from build123d import *

# Parameters (mm, degrees)
SKETCH1_R           = 52.3621
BOSS_EXTRUDE1_DEPTH = 7.06
SKETCH4_R           = 1.7653
SKETCH6_R           = 1.575
CUT_EXTRUDE1_DEPTH  = 7.06
BOSS_EXTRUDE2_DEPTH = 7.06
CUT_EXTRUDE3_DEPTH  = 7.06
CHAMFER17_SIZE      = 4
CHAMFER17_SIZE2     = 2.800830153
CHAMFER18_SIZE      = 4
CHAMFER18_SIZE2     = 2.800830153
CHAMFER19_SIZE      = 4
CHAMFER19_SIZE2     = 2.800830153
CHAMFER20_SIZE      = 4
CHAMFER20_SIZE2     = 2.800830153
CHAMFER21_SIZE      = 4
CHAMFER21_SIZE2     = 2.800830153
CHAMFER25_SIZE      = 4
CHAMFER25_SIZE2     = 2.800830153
CHAMFER26_SIZE      = 4
CHAMFER26_SIZE2     = 2.800830153
CHAMFER39_SIZE      = 4
CHAMFER39_SIZE2     = 2.800830153
CHAMFER40_SIZE      = 4
CHAMFER40_SIZE2     = 2.800830153
CHAMFER42_SIZE      = 4
CHAMFER42_SIZE2     = 2.800830153
CHAMFER43_SIZE      = 4
CHAMFER43_SIZE2     = 2.800830153
CHAMFER44_SIZE      = 4
CHAMFER44_SIZE2     = 2.800830153
CHAMFER45_SIZE      = 4
CHAMFER45_SIZE2     = 2.800830153
CHAMFER46_SIZE      = 4
CHAMFER46_SIZE2     = 2.800830153


with BuildPart() as part:
    # Sketch1 → Boss-Extrude1 (new body)
    with BuildSketch(Plane(origin=(0, 0, 0), x_dir=(1, 0, 0), z_dir=(0, 1, 0))):
        with Locations(Location((0, 0, 0), (0, 0, 270))):
            Circle(SKETCH1_R)
    extrude(amount=BOSS_EXTRUDE1_DEPTH)

    # Sketch4 → Cut-Revolve2 (revolve, cut)
    with BuildSketch(Plane(origin=(0, 0, 0), x_dir=(0, 0, -1), z_dir=(1, 0, 0)), mode=Mode.PRIVATE) as cut_revolve2_sk:
        with Locations((-52.3621, 3.53)):
            Circle(SKETCH4_R)
    revolve(cut_revolve2_sk.sketch.rotate(Axis((0, 3.53, 0), (0, 1, 0)), 180), axis=Axis((0, 3.53, 0), (0, 1, 0)), mode=Mode.SUBTRACT)

    # Sketch6 → Cut-Extrude1 (cut)
    with BuildSketch(Plane(origin=(0, 7.06, 0), x_dir=(1, 0, 0), z_dir=(0, 1, 0))):
        with Locations(Location((0, 0, 0), (0, 0, 270))):
            Circle(SKETCH6_R)
    extrude(amount=-CUT_EXTRUDE1_DEPTH, mode=Mode.SUBTRACT)

    # Sketch7 → Boss-Extrude2 (add)
    with BuildSketch(Plane(origin=(0, 7.06, 0), x_dir=(1, 0, 0), z_dir=(0, 1, 0))):
        with BuildLine():
            Line((-1.173935688, 1.05), (1.173935688, 1.05))
            ThreePointArc((1.173935688, 1.05), (0, 1.575), (-1.173935688, 1.05))
        make_face()
    extrude(amount=-BOSS_EXTRUDE2_DEPTH)

    # Sketch8 → Cut-Extrude3 (cut)
    with BuildSketch(Plane(origin=(0, 7.06, 0), x_dir=(1, 0, 0), z_dir=(0, 1, 0))):
        with BuildLine():
            Line((-44.72135955, 5), (-17.291616466, 5))
            ThreePointArc((-17.291616466, 5), (-16.629831585, 6.888301783), (-15.762553167, 8.691485355))
            Line((-15.762553167, 8.691485355), (-35.158310508, 28.087242696))
            ThreePointArc((-35.158310508, 28.087242696), (-41.574578963, 17.220754456), (-44.72135955, 5))
        make_face()
        with BuildLine():
            Line((-17.291616466, -5), (-44.72135955, -5))
            ThreePointArc((-44.72135955, -5), (-41.574578963, -17.220754456), (-35.158310508, -28.087242696))
            Line((-35.158310508, -28.087242696), (-15.762553167, -8.691485355))
            ThreePointArc((-15.762553167, -8.691485355), (-16.629831585, -6.888301783), (-17.291616466, -5))
        make_face()
        with BuildLine():
            Line((17.291616466, -5), (44.72135955, -5))
            ThreePointArc((44.72135955, -5), (41.574578963, -17.220754456), (35.158310508, -28.087242696))
            Line((35.158310508, -28.087242696), (15.762553167, -8.691485355))
            ThreePointArc((15.762553167, -8.691485355), (16.629831585, -6.888301783), (17.291616466, -5))
        make_face()
        with BuildLine():
            Line((15.762553167, 8.691485355), (35.158310508, 28.087242696))
            ThreePointArc((35.158310508, 28.087242696), (41.574578963, 17.220754456), (44.72135955, 5))
            Line((44.72135955, 5), (17.291616466, 5))
            ThreePointArc((17.291616466, 5), (16.629831585, 6.888301783), (15.762553167, 8.691485355))
        make_face()
        with BuildLine():
            Line((-28.087242696, 35.158310508), (-8.691485355, 15.762553167))
            ThreePointArc((-8.691485355, 15.762553167), (-6.888301783, 16.629831585), (-5, 17.291616466))
            Line((-5, 17.291616466), (-5, 44.72135955))
            ThreePointArc((-5, 44.72135955), (-17.220754456, 41.574578963), (-28.087242696, 35.158310508))
        make_face()
        with BuildLine():
            Line((5, 17.291616466), (5, 44.72135955))
            ThreePointArc((5, 44.72135955), (17.220754456, 41.574578963), (28.087242696, 35.158310508))
            Line((28.087242696, 35.158310508), (8.691485355, 15.762553167))
            ThreePointArc((8.691485355, 15.762553167), (6.888301783, 16.629831585), (5, 17.291616466))
        make_face()
        with BuildLine():
            Line((-28.087242696, -35.158310508), (-8.691485355, -15.762553167))
            ThreePointArc((-8.691485355, -15.762553167), (-6.888301783, -16.629831585), (-5, -17.291616466))
            Line((-5, -17.291616466), (-5, -44.72135955))
            ThreePointArc((-5, -44.72135955), (-17.220754456, -41.574578963), (-28.087242696, -35.158310508))
        make_face()
        with BuildLine():
            Line((5, -17.291616466), (5, -44.72135955))
            ThreePointArc((5, -44.72135955), (17.220754456, -41.574578963), (28.087242696, -35.158310508))
            Line((28.087242696, -35.158310508), (8.691485355, -15.762553167))
            ThreePointArc((8.691485355, -15.762553167), (6.888301783, -16.629831585), (5, -17.291616466))
        make_face()
    extrude(amount=-CUT_EXTRUDE3_DEPTH, mode=Mode.SUBTRACT)

    # Chamfer17
    chamfer17_edges = [part.edges().sort_by_distance(p)[0] for p in [
        (-18.389364025, 7.06, -25.460431837),
        (-25.460431837, 7.06, -18.389364025),
    ]]
    chamfer17_side = [part.faces().sort_by_distance(p)[0] for p in [
        (0, 7.06, -50.881076161),
    ]]
    chamfer(chamfer17_edges, length=CHAMFER17_SIZE, length2=CHAMFER17_SIZE2, reference=chamfer17_side[0])

    # Chamfer18
    chamfer18_edges = [part.edges().sort_by_distance(p)[0] for p in [
        (-18.389364025, 0, -25.460431837),
    ]]
    chamfer18_side = [part.faces().sort_by_distance(p)[0] for p in [
        (0, 0, -50.881076161),
    ]]
    chamfer(chamfer18_edges, length=CHAMFER18_SIZE, length2=CHAMFER18_SIZE2, reference=chamfer18_side[0])

    # Chamfer19
    chamfer19_edges = [part.edges().sort_by_distance(p)[0] for p in [
        (-25.460431837, 0, -18.389364025),
    ]]
    chamfer19_side = [part.faces().sort_by_distance(p)[0] for p in [
        (-19.682698274, 0, -42.107920464),
    ]]
    chamfer(chamfer19_edges, length=CHAMFER19_SIZE, length2=CHAMFER19_SIZE2, reference=chamfer19_side[0])

    # Chamfer20
    chamfer20_edges = [part.edges().sort_by_distance(p)[0] for p in [
        (-31.006488008, 7.06, -5),
        (-31.006488008, 7.06, 5),
    ]]
    chamfer20_side = [part.faces().sort_by_distance(p)[0] for p in [
        (-19.682698274, 7.06, -42.107920464),
    ]]
    chamfer(chamfer20_edges, length=CHAMFER20_SIZE, length2=CHAMFER20_SIZE2, reference=chamfer20_side[0])

    # Chamfer21
    chamfer21_edges = [part.edges().sort_by_distance(p)[0] for p in [
        (18.389364025, 7.06, -25.460431837),
        (5, 7.06, -31.006488008),
        (-5, 7.06, -31.006488008),
        (-25.460431837, 7.06, 18.389364025),
        (31.006488008, 7.06, -5),
        (25.460431837, 7.06, -18.389364025),
        (25.460431837, 7.06, 18.389364025),
        (31.006488008, 7.06, 5),
        (-18.389364025, 7.06, 25.460431837),
        (-5, 7.06, 31.006488008),
        (5, 7.06, 31.006488008),
        (18.389364025, 7.06, 25.460431837),
    ]]
    chamfer21_side = [part.faces().sort_by_distance(p)[0] for p in [
        (2.323352496, 7.06, 0.962148374),
    ]]
    chamfer(chamfer21_edges, length=CHAMFER21_SIZE, length2=CHAMFER21_SIZE2, reference=chamfer21_side[0])

    # Chamfer25
    chamfer25_edges = [part.edges().sort_by_distance(p)[0] for p in [
        (5, 0, -31.006488008),
        (-5, 0, -31.006488008),
    ]]
    chamfer25_side = [part.faces().sort_by_distance(p)[0] for p in [
        (-14.451812174, 0, -8.001356027),
    ]]
    chamfer(chamfer25_edges, length=CHAMFER25_SIZE, length2=CHAMFER25_SIZE2, reference=chamfer25_side[0])

    # Chamfer26
    chamfer26_edges = [part.edges().sort_by_distance(p)[0] for p in [
        (18.389364025, 0, -25.460431837),
        (25.460431837, 0, -18.389364025),
        (31.006488008, 0, -5),
        (31.006488008, 0, 5),
        (25.460431837, 0, 18.389364025),
        (18.389364025, 0, 25.460431837),
    ]]
    chamfer26_side = [part.faces().sort_by_distance(p)[0] for p in [
        (0.962364114, 0, 2.323136756),
    ]]
    chamfer(chamfer26_edges, length=CHAMFER26_SIZE, length2=CHAMFER26_SIZE2, reference=chamfer26_side[0])

    # Chamfer39
    chamfer39_edges = [part.edges().sort_by_distance(p)[0] for p in [
        (16.629831585, 0, 6.888301783),
    ]]
    chamfer39_side = [part.faces().sort_by_distance(p)[0] for p in [
        (-2.671933538, 0, 2.671685429),
    ]]
    chamfer(chamfer39_edges, length=CHAMFER39_SIZE, length2=CHAMFER39_SIZE2, reference=chamfer39_side[0])

    # Chamfer40
    chamfer40_edges = [part.edges().sort_by_distance(p)[0] for p in [
        (16.629831585, 0, -6.888301783),
        (6.888301783, 0, -16.629831585),
        (-6.888301783, 0, -16.629831585),
        (-31.006488008, 0, -5),
        (-31.006488008, 0, 5),
        (-25.460431837, 0, 18.389364025),
        (-18.389364025, 0, 25.460431837),
        (-5, 0, 31.006488008),
        (5, 0, 31.006488008),
    ]]
    chamfer40_side = [part.faces().sort_by_distance(p)[0] for p in [
        (-2.841532186, 0, 2.638527927),
    ]]
    chamfer(chamfer40_edges, length=CHAMFER40_SIZE, length2=CHAMFER40_SIZE2, reference=chamfer40_side[0])

    # Chamfer42
    chamfer42_edges = [part.edges().sort_by_distance(p)[0] for p in [
        (-16.629831585, 0, -6.888301783),
        (-16.629831585, 0, 6.888301783),
        (-6.888301783, 0, 16.629831585),
        (6.888301783, 0, 16.629831585),
    ]]
    chamfer42_side = [part.faces().sort_by_distance(p)[0] for p in [
        (20.502942916, 0, -21.183213354),
    ]]
    chamfer(chamfer42_edges, length=CHAMFER42_SIZE, length2=CHAMFER42_SIZE2, reference=chamfer42_side[0])

    # Chamfer43
    chamfer43_edges = [part.edges().sort_by_distance(p)[0] for p in [
        (-6.888301783, 7.06, -16.629831585),
        (6.888301783, 7.06, -16.629831585),
        (16.629831585, 7.06, -6.888301783),
        (16.629831585, 7.06, 6.888301783),
        (6.888301783, 7.06, 16.629831585),
        (-6.888301783, 7.06, 16.629831585),
        (-16.629831585, 7.06, 6.888301783),
        (-16.629831585, 7.06, -6.888301783),
    ]]
    chamfer43_side = [part.faces().sort_by_distance(p)[0] for p in [
        (22.600241453, 7.06, -21.919971015),
    ]]
    chamfer(chamfer43_edges, length=CHAMFER43_SIZE, length2=CHAMFER43_SIZE2, reference=chamfer43_side[0])

    # Chamfer44
    chamfer44_edges = [part.edges().sort_by_distance(p)[0] for p in [
        (41.574578963, 0, -17.220754456),
    ]]
    chamfer44_side = [part.faces().sort_by_distance(p)[0] for p in [
        (-29.47656378, 0, 0.481023839),
    ]]
    chamfer(chamfer44_edges, length=CHAMFER44_SIZE, length2=CHAMFER44_SIZE2, reference=chamfer44_side[0])

    # Chamfer45
    chamfer45_edges = [part.edges().sort_by_distance(p)[0] for p in [
        (17.220754456, 0, -41.574578963),
        (-17.220754456, 0, -41.574578963),
        (-41.574578963, 0, -17.220754456),
        (-41.574578963, 0, 17.220754456),
        (-17.220754456, 0, 41.574578963),
        (17.220754456, 0, 41.574578963),
        (41.574578963, 0, 17.220754456),
    ]]
    chamfer45_side = [part.faces().sort_by_distance(p)[0] for p in [
        (-1.843064588, 0, 0.763087098),
    ]]
    chamfer(chamfer45_edges, length=CHAMFER45_SIZE, length2=CHAMFER45_SIZE2, reference=chamfer45_side[0])

    # Chamfer46
    chamfer46_edges = [part.edges().sort_by_distance(p)[0] for p in [
        (-41.574578963, 7.06, 17.220754456),
        (-17.220754456, 7.06, 41.574578963),
        (17.220754456, 7.06, 41.574578963),
        (41.574578963, 7.06, 17.220754456),
        (41.574578963, 7.06, -17.220754456),
        (17.220754456, 7.06, -41.574578963),
        (-17.220754456, 7.06, -41.574578963),
        (-41.574578963, 7.06, -17.220754456),
    ]]
    chamfer46_side = [part.faces().sort_by_distance(p)[0] for p in [
        (0.481023839, 7.06, -29.47656378),
    ]]
    chamfer(chamfer46_edges, length=CHAMFER46_SIZE, length2=CHAMFER46_SIZE2, reference=chamfer46_side[0])


solid = part.part
The listing builds one solid part. Answer for the finished solid, in the listing's coordinates (mm). A direction names the side the tool comes from. Round coordinates to 2 decimals unless told otherwise and drop trailing zeros. Write each question's results on one line, items separated by ' | '. Start each with the question number.
1) Find section A-A on z = 20.5. Count the separate pieces of the cut face and the enclosed holes in it, plus the area to 3 significant figures.
2) Straight lines are drawn through the part: probe 1 along X at (y, z) = (3.5, 37.5); probe 2 along Z at (x, y) = (21, 4.75); probe 3 along Z at (x, y) = (30.5, 5.75). For each, find the intervals that lie inside material, in ascending order.
3) Which of the six approach directions +Z, -Z, +X, -X, +Y, -Y give full straight-line access (tool end or side, diameter ignored) to faces 1 (the flat face through (-18.53, 3.54, 25.6)), 2 (the conical face through (-17.58, 5.33, 43.08)), 3 (the flat face through (24.57, 1.42, 20.29))?
4) Each of these flat-tipped pins is pushed along its axis until it touches: pin 1 (1 mm diameter, centred on x = 32.5, y = 2.5, fed in from -Z); pin 2 (1.5 mm diameter, centred on y = 4, z = 10.5, fed in from -X); pin 3 (1.2 mm diameter, centred on y = 3.5, z = -27.5, fed in from +X). Where does it stop, or does it pass through?
Final values:
1) separate pieces: 5 | enclosed holes: 0 | area: 264 mm²
2) probe 1: -33.97 to -24.87, -5 to 5, 24.87 to 33.97 | probe 2: -46.57 to -40.59, -27.08 to -14.92, -4.3 to 4.3, 14.92 to 27.08, 40.59 to 46.57 | probe 3: -42.56 to -35.93, -34.56 to -26.44, -2.87 to 2.87, 26.44 to 34.56, 35.93 to 42.56
3) face 1: +Y, -Y | face 2: +Y | face 3: -Y
4) pin 1: z = -40 | pin 2: x = -50.01 | pin 3: x = 42.85
